```python
from build123d import *

# Parameters (mm, degrees)
F0_R     = 9.5
F1_DEPTH = 2.5
F2_R     = 6.5
F3_DEPTH = 4
F4_R     = 6
F5_DEPTH = 2
F6_R     = 8
F7_DEPTH = 1


with BuildPart() as f1:
    # F0 (on Top) → F1 (new body, symmetric)
    with BuildSketch(Plane.XY):
        Circle(F0_R)
    extrude(amount=F1_DEPTH, both=True)

    # F2 (on face) → F3 (cut)
    with BuildSketch(Plane.XY.offset(2.5)):
        Circle(F2_R)
        with BuildLine():
            ThreePointArc((-0.75, -5.95294), (0, 6), (0.75, -5.95294))
            Line((0.75, -5.95294), (0.75, -5.5))
            Line((0.75, -5.5), (-0.75, -5.5))
            Line((-0.75, -5.5), (-0.75, -5.95294))
        make_face(mode=Mode.SUBTRACT)
        with BuildLine():
            Line((-3.441468, 0.907908), (-2.914973, 0.73684))
            Line((-2.914973, 0.73684), (-2.791366, 1.117262))
            Line((-2.791366, 1.117262), (-3.317861, 1.288331))
            ThreePointArc((-3.317861, 1.288331), (-3.585514, 1.585589), (-3.976773, 1.502424))
            Line((-3.976773, 1.502424), (-4.503268, 1.673493))
            Line((-4.503268, 1.673493), (-4.626875, 1.29307))
            Line((-4.626875, 1.29307), (-4.100379, 1.122002))
            ThreePointArc((-4.100379, 1.122002), (-3.832727, 0.824744), (-3.441468, 0.907908))
        make_face()
        with BuildLine():
            Line((-2.250551, 2.757358), (-1.925159, 2.309494))
            Line((-1.925159, 2.309494), (-1.601552, 2.544608))
            Line((-1.601552, 2.544608), (-1.926944, 2.992472))
            ThreePointArc((-1.926944, 2.992472), (-1.968756, 3.39028), (-2.334174, 3.552975))
            Line((-2.334174, 3.552975), (-2.659566, 4.000839))
            Line((-2.659566, 4.000839), (-2.983173, 3.765725))
            Line((-2.983173, 3.765725), (-2.657781, 3.317861))
            ThreePointArc((-2.657781, 3.317861), (-2.615969, 2.920052), (-2.250551, 2.757358))
        make_face()
        with BuildLine():
            Line((-0.2, 3), (0.2, 3))
            Line((0.2, 3), (0.2, 3.55359))
            ThreePointArc((0.2, 3.55359), (0.4, 3.9), (0.2, 4.24641))
            Line((0.2, 4.24641), (0.2, 4.8))
            Line((0.2, 4.8), (-0.2, 4.8))
            Line((-0.2, 4.8), (-0.2, 4.24641))
            ThreePointArc((-0.2, 4.24641), (-0.4, 3.9), (-0.2, 3.55359))
            Line((-0.2, 3.55359), (-0.2, 3))
        make_face()
        with BuildLine():
            Line((1.926944, 2.992472), (1.601552, 2.544608))
            Line((1.601552, 2.544608), (1.925159, 2.309494))
            Line((1.925159, 2.309494), (2.250551, 2.757358))
            ThreePointArc((2.250551, 2.757358), (2.615969, 2.920052), (2.657781, 3.317861))
            Line((2.657781, 3.317861), (2.983173, 3.765725))
            Line((2.983173, 3.765725), (2.659566, 4.000839))
            Line((2.659566, 4.000839), (2.334174, 3.552975))
            ThreePointArc((2.334174, 3.552975), (1.968756, 3.39028), (1.926944, 2.992472))
        make_face()
        with BuildLine():
            Line((3.317861, 1.288331), (2.791366, 1.117262))
            Line((2.791366, 1.117262), (2.914973, 0.73684))
            Line((2.914973, 0.73684), (3.441468, 0.907908))
            ThreePointArc((3.441468, 0.907908), (3.832727, 0.824744), (4.100379, 1.122002))
            Line((4.100379, 1.122002), (4.626875, 1.29307))
            Line((4.626875, 1.29307), (4.503268, 1.673493))
            Line((4.503268, 1.673493), (3.976773, 1.502424))
            ThreePointArc((3.976773, 1.502424), (3.585514, 1.585589), (3.317861, 1.288331))
        make_face()
    extrude(amount=-F3_DEPTH, mode=Mode.SUBTRACT)

    # F4 (on face) → F5 (cut)
    with BuildSketch(Plane.XY.offset(2.5)):
        Circle(F4_R)
    extrude(amount=-F5_DEPTH, mode=Mode.SUBTRACT)

    # F6 (on face) → F7 (cut)
    with BuildSketch(Plane.XY.offset(2.5)):
        Circle(F6_R)
    extrude(amount=-F7_DEPTH, mode=Mode.SUBTRACT)


solid = f1.part
```
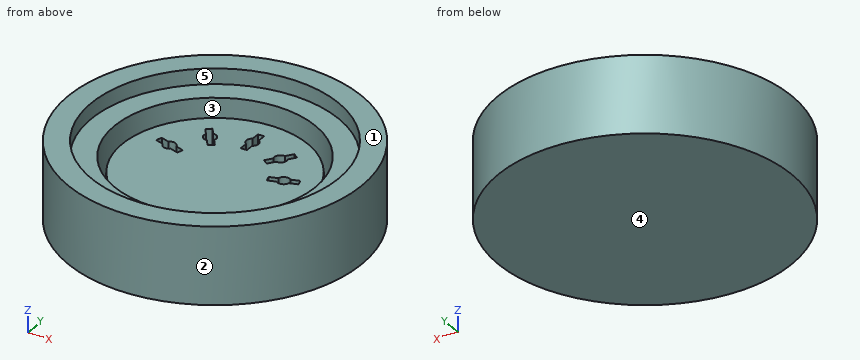
Work out the finished part from the listing and answer in its coordinate system (mm). Face numbers are marked on the shaded views. A direction names the side the tool comes from. Give positions to 0.01 mm unless a question says otherwise; leave off trailing zeros. Loops run counter-clockwise (first coordinate to the right, second up) from the corner with the lowest first, then second, coordinate; pieces in that order, holes last. Notation, with made-up numbers: (37.25, 22.5) -> (42.25, 22.5) arc R18 cw to (42.25, 33.5) -> close; hole circle Ø8 at (28.5, -31). An arc over 180 degrees is marked (long way). Put each result on its own line as item: value. Start each with the question number.
Item 1: The part is cut by section A-A (z = -0.8). State how many separate pieces and enclosed holes the cut face has, then the cut area to 3 significant figures.
Item 2: The part is cut by section C-C (z = 1.15). Give the vertices of the cut face in (x, y), then the cut area to 3 significant figures.
Item 3: Each of these flat-tipped pins is pushed along its axis until it touches: P1, Ø3, axis at x = 5.5, z = 0, coming from the -Y side; P2, Ø4, axis at x = 0, y = 0, coming from the +Z side; P3, Ø0.5, axis at y = -6, z = -1, coming from the -X side. Where does it stop, or does it pass through?
Item 4: The part is cut by section B-B (y = 0). Give the vertices of the cut face in (x, z).
Item 5: The part is cut by section D-D (x = 5.75). Give the vertices of the cut face in (y, z), then the cut area to 3 significant figures.
Item 6: The mould has two halves that part along Y. Classify the marked faces 1, 2 and 3: released by +Y, released by -Y, zero draft, split by the parting line, or undercut.
Item 7: Which of the six approach directions +Z, -Z, +X, -X, +Y, -Y give full straight-line access (tool end or side, diameter ignored) to the marked faces 4 and 5?
Item 8: Find the intervals of material crossed by L1, parallel to Y at x = 0, z = -0.2; L2, parallel to Y at x = 0, z = 2.1; L3, parallel to Y at x = 0, z = 0.8, in increasing order. Write a range as [from, to].
Answers below:
1. separate pieces: 2
1. enclosed holes: 6
1. area: 259 mm2
2. outline: circle Ø19 at (0, 0); hole circle Ø13 at (0, 0)
2. area: 151 mm2
3. P1: y = -8.62
3. P2: z = 0.5
3. P3: x = -7.56
4. outline: (-9.5, -2.5) -> (9.5, -2.5) -> (9.5, 2.5) -> (8, 2.5) -> (8, 1.5) -> (6.5, 1.5) -> (6.5, -1.5) -> (6, -1.5) -> (6, 0.5) -> (-6, 0.5) -> (-6, -1.5) -> (-6.5, -1.5) -> (-6.5, 1.5) -> (-8, 1.5) -> (-8, 2.5) -> (-9.5, 2.5) -> close
5. outline: (-7.56, -2.5) -> (7.56, -2.5) -> (7.56, 2.5) -> (5.56, 2.5) -> (5.56, 1.5) -> (3.03, 1.5) -> (3.03, -1.5) -> (1.71, -1.5) -> (1.71, 0.5) -> (-1.71, 0.5) -> (-1.71, -1.5) -> (-3.03, -1.5) -> (-3.03, 1.5) -> (-5.56, 1.5) -> (-5.56, 2.5) -> (-7.56, 2.5) -> close
5. area: 53.2 mm2
6. face 1: zero draft
6. face 2: split by the parting line
6. face 3: undercut
7. face 4: -Z, +X, -X, +Y, -Y
7. face 5: +Z
8. L1: [-9.5, -6.5], [-5.5, 3], [4.8, 6], [6.5, 9.5]
8. L2: [-9.5, -8], [8, 9.5]
8. L3: [-9.5, -6.5], [6.5, 9.5]
